Autodesk Inventor part; units mm, degrees
ref_plane "YZ Plane" through (0, 0, 0) normal (1, 0, 0) x (0, 1, 0)
ref_plane "XZ Plane" through (0, 0, 0) normal (0, 1, 0) x (-1, 0, 0)
ref_plane "XY Plane" through (0, 0, 0) normal (0, 0, 1) x (1, 0, 0)
sketch "Skizze1" plane through (0, 0, 0) normal (0, 0, 1) x (1, 0, 0)
  line L0 (0, 0) -> (52, 0)
  line L1 (52, 0) -> (52, -84)
  line L2 (52, -84) -> (0, -84)
  line L3 (0, -84) -> (0, 0)
  dimension "d0" = 52
  dimension "d1" = 84
extrude "Extrusion1" add sketch "Skizze1" along normal blind 2
sketch "Skizze2" plane through (0, 0, 2) normal (0, 0, 1) x (1, 0, 0)
  line L0 (48, -8) -> (4, -8)
  line L1 (4, -8) -> (4, -76)
  line L2 (4, -76) -> (48, -76)
  line L3 (48, -76) -> (48, -8)
  line L4 (52, 0) -> (0, 0)
  line L5 (52, -84) -> (52, 0)
  line L6 (0, -84) -> (52, -84)
  point P0 (26, -8)
  point P1 (26, 0)
  dimension "d4" = 4
  dimension "d5" = 8
  dimension "d6" = 8
extrude "Extrusion2" add sketch "Skizze2" along normal blind 2
sketch "Skizze3" plane through (4, -8, 2) normal (0, 1, 0) x (1, 0, 0)
  line L0 (48, 2) -> (-4, 2)
  line L1 (-4, 2) -> (-4, 0)
  line L2 (48, 0) -> (-4, 0)
  line L3 (48, 2) -> (48, 0)
  line L4 (44, -2) -> (0, -2)
  line L5 (32, 0) -> (12, 0)
  line L6 (12, 0) -> (12, -2)
  line L7 (12, -2) -> (32, -2)
  line L8 (32, -2) -> (32, 0)
  line L9 (44, 0) -> (44, -2)
  point P0 (44, -1)
  point P1 (32, -2)
  point P2 (12, 0)
  dimension "d9" = 20
  dimension "d10" = 12
extrude "Extrusion3" cut sketch "Skizze3" against normal through all contours L2 L8 L4 L6
sketch "Skizze4" plane through (0, 0, 2) normal (0, 0, 1) x (1, 0, 0)
  line L0 (52, 0) -> (0, 0)
  line L1 (0, -84) -> (52, -84)
  point P0 (26, -4)
  point P1 (26, -80)
  point P2 (26, 0)
  dimension "d20" = 4
  dimension "d21" = 4
hole "Bohrung1" at (26, -4, 2) at (26, -80, 2) direction (0, 0, -1) diameter 4 depth 2
equation "\"d6\" = d5"
properties part number "1011" material "Aluminum 6061-AHC"
For this review, take the finished solid that the model builds, in its own axes (mm). A direction names the side the tool comes from. Round coordinates to 2 decimals unless told otherwise and drop trailing zeros. Write each loop counter-clockwise with the first axis right and the second up, starting at its lowest first coordinate (ties: lowest second). Pieces come first, ordered by that corner, then holes. Notation, with made-up numbers: (6.25, 78.5) - (54.25, 78.5) arc R27 ccw to (54.25, 99.5) - close; hole circle Ø4 at (56.5, 26.5). An arc over 180 degrees is marked (long way). Write item = value, one per line. Start each with the question number.
1. For pin 1 Ø0.6 at (x, z) = (7.5, 2.5) entering from +Y; pin 2 Ø1.5 at (y, z) = (-40, 3.5) entering from +X; pin 3 Ø8 at (x, y) = (37, -21.5) entering from -Z; pin 4 Ø3.5 at (x, y) = (26, -80) entering from -Z, all flat-tipped, find the tip position at first contact; note any pin that passes through.
2. Wall thickness on L1, parallel to Y at x = 26, z = 0.4; L2, parallel to X at y = -29, z = 2.95; L3, parallel to X at y = -80, z = 0.75: over which ranges is each line inside the solid? List them lowest first.
3. Consider section B-B on x = 26. State the section outline as (y, z) points.
4. Consider section C-C on y = -4. State the section outline as (x, z) points.
5. Draft analysis for pull direction Y (two halves, no side actions). For faces 1 (the face through (25.399, -81.908, 0.986)), 2 (the face through (26, 0, 1)), 3 (the face through (26, -41, 2)), state which applies: released by +Y, released by -Y, zero draft, split by the parting line, or undercut.
6. Consider section D-D on y = -14. State the section outline as (x, z) points, plus the area to 3 significant figures.
7. Consider section A-A on z = 3. State the section outline as (x, y) points, plus the area to 3 significant figures.
8. For faces 4 (the face through (10, -76, 3)), 5 (the face through (10, -8, 3)), 6 (the face through (36, -42, 3)), 7 (the face through (48, -42, 3)), list the 3-axis set-ups (+Z, -Z, +X, -X, +Y, -Y) from which the entire face can be reached by the end or side of a thin tool; tool diameter is ignored.
Evaluation:
q1.pin_1 = -8
q1.pin_2 = 48
q1.pin_3 = 0
q1.pin_4 = through
q2.L1 = -84 to -82, -78 to -6, -2 to 0
q2.L2 = 4 to 16, 36 to 48
q2.L3 = 0 to 24, 28 to 52
q3.outline = (-84, 0) - (-82, 0) - (-82, 2) - (-84, 2) - close; (-78, 0) - (-6, 0) - (-6, 2) - (-78, 2) - close; (-2, 0) - (0, 0) - (0, 2) - (-2, 2) - close
q4.outline = (0, 0) - (24, 0) - (24, 2) - (0, 2) - close; (28, 0) - (52, 0) - (52, 2) - (28, 2) - close
q5.face_1 = undercut
q5.face_2 = released by +Y
q5.face_3 = zero draft
q6.outline = (0, 0) - (52, 0) - (52, 2) - (48, 2) - (48, 4) - (36, 4) - (36, 2) - (16, 2) - (16, 4) - (4, 4) - (4, 2) - (0, 2) - close
q6.area = 152 mm2
q7.outline = (4, -76) - (16, -76) - (16, -8) - (4, -8) - close; (36, -76) - (48, -76) - (48, -8) - (36, -8) - close
q7.area = 1,630 mm2
q8.face_4 = +Z, +X, -X, -Y
q8.face_5 = +Z, +X, -X, +Y
q8.face_6 = +Z, +Y, -Y
q8.face_7 = +Z, +X, +Y, -Y
